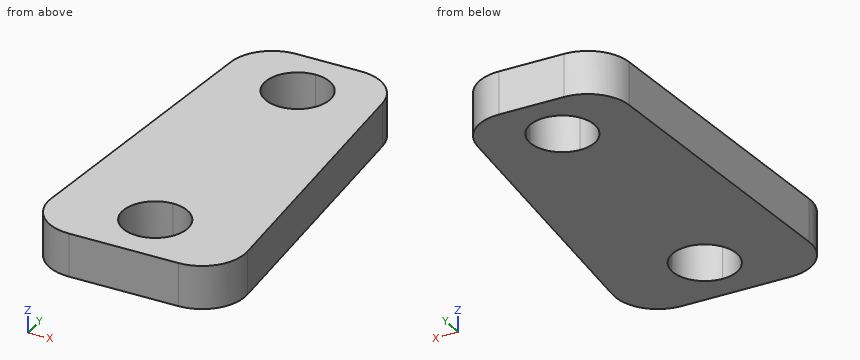
from build123d import *

# Parameters (mm, degrees)
BOSS_EXTRUDE1_DEPTH = 3.175


with BuildPart() as part:
    # Sketch1 → Boss-Extrude1 (new body)
    with BuildSketch(Plane.XY):
        with BuildLine():
            Line((0, 135.477250085), (0, 137.244666667))
            Line((0, 137.244666667), (-2.377569082, 137.244666667))
            ThreePointArc((-2.377569082, 137.244666667), (-4.534821542, 136.399234614), (-5.543217073, 134.313178051))
            Line((-5.543217073, 134.313178051), (-7.164909381, 113.231178051))
            ThreePointArc((-7.164909381, 113.231178051), (-6.328829337, 110.830414206), (-3.999261389, 109.812666667))
            Line((-3.999261389, 109.812666667), (0, 109.812666667))
            Line((0, 109.812666667), (0, 111.664750085))
            ThreePointArc((0, 111.664750085), (-2.38125, 114.046000085), (0, 116.427250085))
            Line((0, 116.427250085), (0, 130.714750085))
            ThreePointArc((0, 130.714750085), (-2.38125, 133.096000085), (0, 135.477250085))
        make_face()
        with BuildLine():
            Line((7.164909381, 113.231178051), (5.543217073, 134.313178051))
            ThreePointArc((5.543217073, 134.313178051), (4.534821542, 136.399234614), (2.377569082, 137.244666667))
            Line((2.377569082, 137.244666667), (0, 137.244666667))
            Line((0, 137.244666667), (0, 135.477250085))
            ThreePointArc((0, 135.477250085), (1.683798023, 134.779798107), (2.38125, 133.096000085))
            ThreePointArc((2.38125, 133.096000085), (1.683798023, 131.412202062), (0, 130.714750085))
            Line((0, 130.714750085), (0, 116.427250085))
            ThreePointArc((0, 116.427250085), (1.683798023, 115.729798107), (2.38125, 114.046000085))
            ThreePointArc((2.38125, 114.046000085), (1.683798023, 112.362202062), (0, 111.664750085))
            Line((0, 111.664750085), (0, 109.812666667))
            Line((0, 109.812666667), (3.999261389, 109.812666667))
            ThreePointArc((3.999261389, 109.812666667), (6.328829337, 110.830414206), (7.164909381, 113.231178051))
        make_face()
    extrude(amount=BOSS_EXTRUDE1_DEPTH)


solid = part.part
Geometry: final body of the model. Coordinates: model frame, mm. Round coordinates to 2 decimals unless told otherwise and drop trailing zeros. Write each loop counter-clockwise with the first axis right and the second up, starting at its lowest first coordinate (ties: lowest second). Pieces come first, ordered by that corner, then holes. Notation, with made-up numbers: M 46.25,41.5 L 101.25,41.5 A7 ccw 101.25,54.5 Z; hole C 8.5,69 d9. An arc over 180 degrees is marked long. Write item = value, one per line.
Item 1: Section query B-B on y = 115.5. Return loops of the section in (x, z) (3 decimals).
Findings:
outline = M -6.99,0 L -1.886,0 L -1.886,3.175 L -6.99,3.175 Z; M 1.886,0 L 6.99,0 L 6.99,3.175 L 1.886,3.175 Z
Item 2: Section query C-C on x = 4.75. Return loops of the section in (y, z) (3 decimals).
Findings:
outline = M 109.903,0 L 136.18,0 L 136.18,3.175 L 109.903,3.175 Z
Item 3: Material intervals for line 1 along Y through (x, z) = (1.25, 2.9); line 2 along Y through (x, z) = (-0.5, 2.5); line 3 along X through (y, z) = (124.25, 0.45), sorted ascending. Write a range as [from, to].
Findings:
line_1 = [109.81, 112.02], [116.07, 131.07], [135.12, 137.24]
line_2 = [109.81, 111.72], [116.37, 130.77], [135.42, 137.24]
line_3 = [-6.32, 6.32]
Item 4: Section query A-A on z = 2.5. State how many separate pieces and enclosed holes the cut face has, then the cut area to 3 significant figures.
Findings:
separate_pieces = 1
enclosed_holes = 2
area = 305 mm^2
Item 5: Section query D-D on y = 121.5. Return loops of the section in (x, z) (3 decimals), then the cut area to 3 significant figures.
Findings:
outline = M -6.529,0 L 6.529,0 L 6.529,3.175 L -6.529,3.175 Z
area = 41.5 mm^2
